```python
from build123d import *

# Parameters (mm, degrees)
BOSS_EXTRU_1_DEPTH = 5
BOSS_EXTRU_2_DEPTH = 5
CONG_1_R           = 0.1


with BuildPart() as part:
    # Esquisse1 → Boss.-Extru.1 (new body)
    with BuildSketch(Plane(origin=(0, 0, 0), x_dir=(1, 0, 0), z_dir=(0, 1, 0))):
        with BuildLine():
            Line((19.464682141, -16.403463282), (-20.535317859, -16.403463282))
            Line((-20.535317859, -16.403463282), (-20.968330561, -16.653463282))
            Line((-20.968330561, -16.653463282), (-45.035317859, -58.338708067))
            ThreePointArc((-45.035317859, -58.338708067), (-45.597740084, -58.57167098), (-45.968330561, -58.088708067))
            Line((-45.968330561, -58.088708067), (-45.968330561, -4.954733471))
            ThreePointArc((-45.968330561, -4.954733471), (-0.535317859, 40.478279231), (44.897694842, -4.954733471))
            Line((44.897694842, -4.954733471), (44.897694842, -58.088708067))
            ThreePointArc((44.897694842, -58.088708067), (44.527104365, -58.57167098), (43.964682141, -58.338708067))
            Line((43.964682141, -58.338708067), (19.897694842, -16.653463282))
            Line((19.897694842, -16.653463282), (19.464682141, -16.403463282))
        make_face()
    extrude(amount=BOSS_EXTRU_1_DEPTH)

    # Esquisse3 → Boss.-Extru.2 (add)
    with BuildSketch(Plane.XZ):
        with BuildLine():
            Line((-17.908394248, 19.818657818), (-17.084754205, 18.533779345))
            Line((-17.084754205, 18.533779345), (-33.79214282, 7.957290442))
            ThreePointArc((-33.79214282, 7.957290442), (-34.004929664, 7.395599901), (-33.524704444, 7.034825396))
            Line((-33.524704444, 7.034825396), (33.003204413, 7.034825396))
            ThreePointArc((33.003204413, 7.034825396), (33.484427413, 7.399088796), (33.264482707, 7.961127698))
            Line((33.264482707, 7.961127698), (16.014118486, 18.533779345))
            Line((16.014118486, 18.533779345), (16.837758529, 19.818657818))
            Line((16.837758529, 19.818657818), (17.939784376, 19.182402899))
            Line((17.939784376, 19.182402899), (17.287895758, 21.086077969))
            Line((17.287895758, 21.086077969), (15.515071867, 22.109618319))
            Line((15.515071867, 22.109618319), (13.540496587, 21.722332888))
            Line((13.540496587, 21.722332888), (14.642522434, 21.086077969))
            Line((14.642522434, 21.086077969), (13.941605057, 19.730345531))
            Line((13.941605057, 19.730345531), (-15.012240776, 19.730345531))
            Line((-15.012240776, 19.730345531), (-15.713158153, 21.086077969))
            Line((-15.713158153, 21.086077969), (-14.611132306, 21.722332888))
            Line((-14.611132306, 21.722332888), (-16.585707586, 22.109618319))
            Line((-16.585707586, 22.109618319), (-18.358531477, 21.086077969))
            Line((-18.358531477, 21.086077969), (-19.010420095, 19.182402899))
            Line((-19.010420095, 19.182402899), (-17.908394248, 19.818657818))
        make_face()
    extrude(amount=BOSS_EXTRU_2_DEPTH)

    # Congé1
    cong_1_edges = [part.edges().sort_by_distance(p)[0] for p in [
        (16.837758529, -2.5, 19.818657818),
        (17.939784376, -2.5, 19.182402899),
        (17.287895758, -2.5, 21.086077969),
        (15.515071867, -2.5, 22.109618319),
        (13.540496587, -2.5, 21.722332888),
        (13.941605057, -2.5, 19.730345531),
        (-15.012240776, -2.5, 19.730345531),
        (-15.713158153, -2.5, 21.086077969),
        (-14.611132306, -2.5, 21.722332888),
        (-16.585707586, -2.5, 22.109618319),
        (-18.358531477, -2.5, 21.086077969),
        (-19.010420095, -2.5, 19.182402899),
        (-17.908394248, -2.5, 19.818657818),
        (-17.084754205, -2.5, 18.533779345),
    ]]
    fillet(cong_1_edges, radius=CONG_1_R)


solid = part.part
```
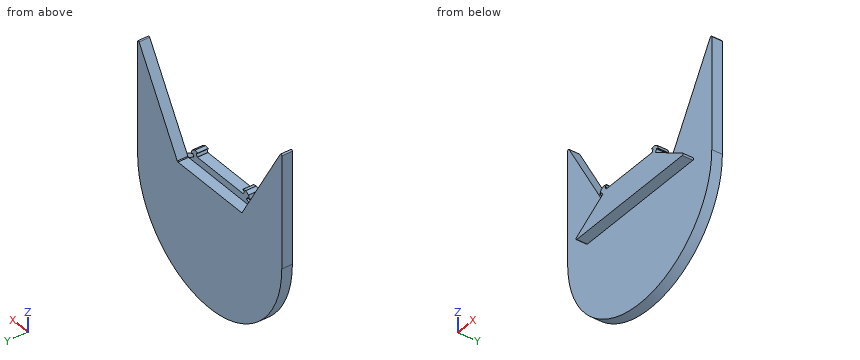
Model file for the job. Use its own axes, mm. Coordinates: 2 decimals unless noted, no trailing zeros. Loops run counter-clockwise (first coordinate to the right, second up) from the corner with the lowest first, then second, coordinate; pieces in that order, holes last. Notation, with made-up numbers: (75.5, -30.75) - (127.5, -30.75) arc R22 cw to (127.5, -9.75) - close; hole circle Ø5 at (64.25, 42). An arc over 180 degrees is marked (long way). Answer as a JSON object with one key per item and string values. Group by question number.
(1) Probe line 1 along Y through (x, z) = (-2, -18); line 2 along Z through (x, y) = (5, -3.5); line 3 along X through (y, z) = (2.25, 51.5). List the from-to ranges inside material, lowest first.
(2) Cut at D-D (z = 52). Give the cut face in (x, y), then the cut area to 3 significant figures.
(3) Cut at A-A (z = 28). Give the cut face in (x, y).
(4) Flat gauge pins, fed straight in: pin 1 (4 mm diameter, centred on x = -7, y = -3, fed in from +Z); pin 2 (12 mm diameter, centred on x = -4, z = -3.5, fed in from -Y); pin 3 (5.5 mm diameter, centred on x = -1, y = -2.5, fed in from -Z); pin 4 (3 mm diameter, centred on x = -31, z = 38.5, fed in from -Y). Where does each tip first touch, or does it go through?
(5) Cut at C-C (x = -32). Give the cut face in (y, z), then the cut area to 3 significant figures.
Geometry says:
{
 "1": {"line 1": "y = 0 to 5", "line 2": "z = 7.03 to 19.73", "line 3": "x = -45.97 to -41.09, 40.02 to 44.9"},
 "2": {"outline": "(-45.97, 0) - (-41.38, 0) - (-41.38, 5) - (-45.97, 5) - close; (40.31, 0) - (44.9, 0) - (44.9, 5) - (40.31, 5) - close", "area": "45.9 mm^2"},
 "3": {"outline": "(-45.97, 0) - (-27.52, 0) - (-27.52, 5) - (-45.97, 5) - close; (26.45, 0) - (44.9, 0) - (44.9, 5) - (26.45, 5) - close"},
 "4": {"pin 1": "stops at z = 19.73", "pin 2": "stops at y = 0", "pin 3": "stops at z = -40.48", "pin 4": "passes through"},
 "5": {"outline": "(-5, 7.03) - (0, 7.03) - (0, -27.82) - (5, -27.82) - (5, 35.76) - (0, 35.76) - (0, 9.09) - (-5, 9.09) - close", "area": "328 mm^2"}
}
